```python
from build123d import *

# Parameters (mm, degrees)
CROQUIS1_W              = 55
CROQUIS1_H              = 55
CROQUIS1_R              = 1.5
SALIENTE_EXTRUIR1_DEPTH = 5
CROQUIS2_W              = 65
CROQUIS2_H              = 65
CROQUIS2_W_2            = 55
CROQUIS2_H_2            = 55
SALIENTE_EXTRUIR2_DEPTH = 5


with BuildPart() as part:
    # Croquis1 → Saliente-Extruir1 (new body)
    with BuildSketch(Plane(origin=(0, 0, 0), x_dir=(1, 0, 0), z_dir=(0, 1, 0))):
        with Locations((27.5, 27.5)):
            Rectangle(CROQUIS1_W, CROQUIS1_H)
        with Locations(Location((1.75, 42.5, 0), (0, 0, 270))):
            Circle(CROQUIS1_R, mode=Mode.SUBTRACT)
        with Locations(Location((1.75, 12.5, 0), (0, 0, 270))):
            Circle(CROQUIS1_R, mode=Mode.SUBTRACT)
        with Locations(Location((53.25, 42.5, 0), (0, 0, 90))):
            Circle(CROQUIS1_R, mode=Mode.SUBTRACT)
        with Locations(Location((53.25, 12.5, 0), (0, 0, 90))):
            Circle(CROQUIS1_R, mode=Mode.SUBTRACT)
        Polygon((13.5, 13.5), (27.1, 13.5), (27.1, 10.5), (27.9, 10.5), (27.9, 13.5), (41.5, 13.5), (41.5, 27.1), (44.5, 27.1), (44.5, 27.9), (41.5, 27.9), (41.5, 41.5), (27.9, 41.5), (27.9, 44.5), (27.1, 44.5), (27.1, 41.5), (13.5, 41.5), (13.5, 27.9), (10.5, 27.9), (10.5, 27.1), (13.5, 27.1), align=None, mode=Mode.SUBTRACT)
    extrude(amount=SALIENTE_EXTRUIR1_DEPTH)

    # Croquis2 → Saliente-Extruir2 (add)
    with BuildSketch(Plane(origin=(0, 5, 0), x_dir=(1, 0, 0), z_dir=(0, 1, 0))):
        with Locations((27.5, 27.5)):
            Rectangle(CROQUIS2_W, CROQUIS2_H)
        with Locations((27.5, 27.5)):
            Rectangle(CROQUIS2_W_2, CROQUIS2_H_2, mode=Mode.SUBTRACT)
    extrude(amount=-SALIENTE_EXTRUIR2_DEPTH)


solid = part.part
```
Build history of the part. All positions in model axes, mm. A direction names the side the tool comes from. Coordinates: 2 decimals unless noted, no trailing zeros. Order: outer loops, then holes, each group sorted by start corner. A loop starts at its lowest first (then second) coordinate and runs counter-clockwise, first axis right, second up. Notation, with made-up numbers: M 62,-8 L 76,-8 A29 ccw 76,20 Z; hole C -30.5,13.5 d3. An arc over 180 degrees is marked long. One line per question, with ' | ' between items. Start each with the question number.
1. Cut at C-C (z = -12.5). Write the cut outline in (x, y), plus the area to 3 significant figures.
2. Cut at D-D (x = 1.75). Write the cut outline in (y, z).
3. Cut at B-B (y = 2.7). Write the cut outline in (x, z).
4. Cut at A-A (x = 38). Write the cut outline in (y, z), plus the area to 3 significant figures.
5. Mould opens along Z. For faces 3 (the face through (27, 3, -60)), 4 (the face through (20, 5, -42)), 5 (the face through (27.1, 2, -12)) say: +Z half, -Z half, draft (parallel to the pull), parting line (faces both ways), or undercut.
6. Tool access for faces 1 (the face through (-5, 3, -27)), 2 (the face through (13.5, 2, -20)): list every direction of +Z, -Z, +X, -X, +Y, -Y with a clear straight run to the whole face (end or side of a thin tool).
7. Flat gauge pin, fed straight in: P1, Ø1.8, axis at x = 1.75, z = -42.5, coming from the -Y side. Where does the tip first touch, or does it go through?
8. Wall check: line 1 along X through (y, z) = (1.95, -42.5); line 2 along Z through (x, y) = (53.25, 2.05); line 3 along Z through (x, y) = (19, 1.5). Give the ranges that are in metal, low to high. Write a range as [from, to].
The answers:
1) outline: M -5,0 L 0.25,0 L 0.25,5 L -5,5 Z; M 3.25,0 L 27.1,0 L 27.1,5 L 3.25,5 Z; M 27.9,0 L 51.75,0 L 51.75,5 L 27.9,5 Z; M 54.75,0 L 60,0 L 60,5 L 54.75,5 Z | area: 291 mm2
2) outline: M 0,-60 L 5,-60 L 5,-44 L 0,-44 Z; M 0,-41 L 5,-41 L 5,-14 L 0,-14 Z; M 0,-11 L 5,-11 L 5,5 L 0,5 Z
3) outline: M -5,-60 L 60,-60 L 60,5 L -5,5 Z; hole C 1.75,-42.5 d3; hole C 1.75,-12.5 d3; hole M 10.5,-27.9 L 13.5,-27.9 L 13.5,-41.5 L 27.1,-41.5 L 27.1,-44.5 L 27.9,-44.5 L 27.9,-41.5 L 41.5,-41.5 L 41.5,-27.9 L 44.5,-27.9 L 44.5,-27.1 L 41.5,-27.1 L 41.5,-13.5 L 27.9,-13.5 L 27.9,-10.5 L 27.1,-10.5 L 27.1,-13.5 L 13.5,-13.5 L 13.5,-27.1 L 10.5,-27.1 Z; hole C 53.25,-42.5 d3; hole C 53.25,-12.5 d3
4) outline: M 0,-60 L 5,-60 L 5,-41.5 L 0,-41.5 Z; M 0,-13.5 L 5,-13.5 L 5,5 L 0,5 Z | area: 185 mm2
5) face 3: -Z half | face 4: draft | face 5: undercut
6) face 1: +Z, -Z, -X, +Y, -Y | face 2: +Y, -Y
7) P1: passes through
8) line 1: x = [-5, 0.25], [3.25, 27.1], [27.9, 51.75], [54.75, 60] | line 2: z = [-60, -44], [-41, -14], [-11, 5] | line 3: z = [-60, -41.5], [-13.5, 5]
